from build123d import *

# Parameters (mm, degrees)
SKETCH1_R           = 62.5
BOSS_EXTRUDE1_DEPTH = 23
SKETCH2_R           = 7.5
CUT_EXTRUDE1_DEPTH  = 92.331812639
SKETCH3_R           = 6.402299088
CUT_EXTRUDE2_DEPTH  = 17.51881
CIRPATTERN1_START   = 5.481190123
CIRPATTERN1_DEPTH   = 17.518809877


# Read off the part's stored shape, not the designer's step: CirPattern1
with BuildPart() as part:
    # Sketch1 → Boss-Extrude1 (new body)
    with BuildSketch(Plane(origin=(0, 0, 0), x_dir=(1, 0, 0), z_dir=(0, 1, 0))):
        with Locations(Location((0, 0, 0), (0, 0, 270))):
            Circle(SKETCH1_R)
    extrude(amount=BOSS_EXTRUDE1_DEPTH)

    # Sketch2 → Cut-Extrude1 (cut, through all)
    with BuildSketch(Plane(origin=(0, 0, 0), x_dir=(1, 0, 0), z_dir=(0, 1, 0))):
        with Locations(Location((0, 0, 0), (0, 0, 270))):
            Circle(SKETCH2_R)
    extrude(amount=CUT_EXTRUDE1_DEPTH, mode=Mode.SUBTRACT)

    # Sketch3 → Cut-Extrude2 (cut)
    with BuildSketch(Plane(origin=(0, 23, 0), x_dir=(1, 0, 0), z_dir=(0, 1, 0))):
        with Locations(Location((-16.05131074, 0, 0), (0, 0, 270))):
            Circle(SKETCH3_R)
    extrude(amount=-CUT_EXTRUDE2_DEPTH, mode=Mode.SUBTRACT)

    # CirPattern1 outline → CirPattern1 (cut)
    with BuildSketch(Plane(origin=(0, 0, 0), x_dir=(1, 0, 0), z_dir=(0, 1, 0)).offset(CIRPATTERN1_START)):
        with BuildLine():
            ThreePointArc((4.98422694, -12.032988277), (0, -9.649011652), (-4.98422694, -12.032988277))
            ThreePointArc((-4.98422694, -12.032988277), (-6.822881571, -6.822881571), (-12.032988277, -4.98422694))
            ThreePointArc((-12.032988277, -4.98422694), (-13.60125695, -5.914953088), (-15.368313134, -6.365763731))
            ThreePointArc((-15.368313134, -6.365763731), (-15.877099771, -15.877099771), (-6.365763731, -15.368313134))
            ThreePointArc((-6.365763731, -15.368313134), (0, -22.453609827), (6.365763731, -15.368313134))
            ThreePointArc((6.365763731, -15.368313134), (15.877099771, -15.877099771), (15.368313134, -6.365763731))
            ThreePointArc((15.368313134, -6.365763731), (22.453609827, 0), (15.368313134, 6.365763731))
            ThreePointArc((15.368313134, 6.365763731), (15.877099771, 15.877099771), (6.365763731, 15.368313134))
            ThreePointArc((6.365763731, 15.368313134), (0, 22.453609827), (-6.365763731, 15.368313134))
            ThreePointArc((-6.365763731, 15.368313134), (-15.877099771, 15.877099771), (-15.368313134, 6.365763731))
            ThreePointArc((-15.368313134, 6.365763731), (-13.60125695, 5.914953088), (-12.032988277, 4.98422694))
            ThreePointArc((-12.032988277, 4.98422694), (-6.822881571, 6.822881571), (-4.98422694, 12.032988277))
            ThreePointArc((-4.98422694, 12.032988277), (0, 9.649011652), (4.98422694, 12.032988277))
            ThreePointArc((4.98422694, 12.032988277), (6.822881571, 6.822881571), (12.032988277, 4.98422694))
            ThreePointArc((12.032988277, 4.98422694), (9.649011652, 0), (12.032988277, -4.98422694))
            ThreePointArc((12.032988277, -4.98422694), (6.822881571, -6.822881571), (4.98422694, -12.032988277))
        make_face()
    extrude(amount=CIRPATTERN1_DEPTH, mode=Mode.SUBTRACT)


solid = part.part
Design review of the part built by this model. Coordinates are the model's own, in mm. A direction names the side the tool comes from. Round coordinates to 2 decimals unless told otherwise and drop trailing zeros. Write each loop counter-clockwise with the first axis right and the second up, starting at its lowest first coordinate (ties: lowest second). Pieces come first, ordered by that corner, then holes.
Item 1: Consider section D-D on y = 2.75. Give the boundary of the cut face in (x, z), and give its area (3 significant figures).
Item 2: Consider section A-A on x = 0. Give the boundary of the cut face in (y, z), and give its area (3 significant figures).
Item 3: For pin 1 Ø16.5 at (x, z) = (16.05, 0) entering from +Y; pin 2 Ø5 at (y, z) = (3, 43.5) entering from +X; pin 3 Ø1 at (x, y) = (-1.5, 19.5) entering from -Z; pin 4 Ø2 at (y, z) = (16, 41) entering from +X, all flat-tipped, find the tip position at first contact; note any pin that passes through.
Item 4: Draft analysis for pull direction X (two halves, no side actions). For faces 1 (the flat face through (-27, 23, -1)), 2 (the cylindrical face through (6.88, 14.118, 6.767)), state which applies: released by +X, released by -X, zero draft, split by the parting line, or undercut.
Item 5: For faces 3 (the cylindrical face through (-0.08, 14.12, -9.65)), 4 (the flat face through (-13, 0, -1)), list the 3-axis set-ups (+Z, -Z, +X, -X, +Y, -Y) from which the entire face can be reached by the end or side of a thin tool; tool diameter is ignored.
Item 6: Consider section B-B on z = 0. Give the boundary of the cut face in (x, y), and give its area (3 significant figures).
Item 7: Consider section C-C on y = 16. Give the boundary of the cut face in (x, z).
Item 8: Wall thickness on L1, parallel to X at y = 12.75, z = -4.5; L2, parallel to Z at x = 11.5, y = 8.75; L3, parallel to Y at x = 16.5, z = -5: over which ranges is each line inside the solid? List them lowest first.
Check values:
1. outline: circle Ø125 at (0, 0); hole circle Ø15 at (0, 0)
1. area: 12,100 mm2
2. outline: (0, -62.5) - (23, -62.5) - (23, -22.45) - (5.48, -22.45) - (5.48, -9.65) - (23, -9.65) - (23, -7.5) - (0, -7.5) - close; (0, 7.5) - (23, 7.5) - (23, 9.65) - (5.48, 9.65) - (5.48, 22.45) - (23, 22.45) - (23, 62.5) - (0, 62.5) - close
2. area: 2,080 mm2
3. pin 1: stops at y = 23
3. pin 2: stops at x = 47.17
3. pin 3: stops at z = -62.49
3. pin 4: stops at x = 48.02
4. face 1: zero draft
4. face 2: undercut
5. face 3: +Y
5. face 4: +Z, -Z, +X, -X, -Y
6. outline: (-62.5, 0) - (-7.5, 0) - (-7.5, 23) - (-9.65, 23) - (-9.65, 5.48) - (-22.45, 5.48) - (-22.45, 23) - (-62.5, 23) - close; (7.5, 0) - (62.5, 0) - (62.5, 23) - (22.45, 23) - (22.45, 5.48) - (9.65, 5.48) - (9.65, 23) - (7.5, 23) - close
6. area: 2,080 mm2
7. outline: circle Ø125 at (0, 0); (-12.03, -4.98) arc R6.4 cw to (-4.98, -12.03) arc R6.4 cw to (4.98, -12.03) arc R6.4 cw to (12.03, -4.98) arc R6.4 cw to (12.03, 4.98) arc R6.4 cw to (4.98, 12.03) arc R6.4 cw to (-4.98, 12.03) arc R6.4 cw to (-12.03, 4.98) arc R6.4 cw to start; hole (-15.37, -6.37) arc R6.4 ccw (long way) to (-6.37, -15.37) arc R6.4 ccw (long way) to (6.37, -15.37) arc R6.4 ccw (long way) to (15.37, -6.37) arc R6.4 ccw (long way) to (15.37, 6.37) arc R6.4 ccw (long way) to (6.37, 15.37) arc R6.4 ccw (long way) to (-6.37, 15.37) arc R6.4 ccw (long way) to (-15.37, 6.37) arc R6.4 ccw (long way) to start; hole circle Ø15 at (0, 0)
8. L1: x = -62.34 to -20.61, -11.5 to -6, 6 to 11.5, 20.61 to 62.34
8. L2: z = -61.43 to -17.75, -4.95 to -4.5, 4.5 to 4.95, 17.75 to 61.43
8. L3: y = 0 to 5.48
